Can you work these out from the model? Positions are in its coordinate system, mm. A direction names the side the tool comes from. Coordinates: 2 decimals unless noted, no trailing zeros. Write each loop counter-clockwise with the first axis right and the second up, starting at its lowest first coordinate (ties: lowest second). Pieces come first, ordered by that corner, then holes. Notation, with made-up numbers: M 8.25,51 L 13.25,51 A10 ccw 13.25,63 Z; hole C 48,-3.75 d10. An arc over 180 degrees is marked long. Use one line per item in the form item = value. Start each with the question number.
```python
from build123d import *

# Parameters (mm, degrees)
SKETCH003_R   = 292.1
SKETCH003_R_2 = 6.35
PAD003_DEPTH  = 19.05
SKETCH004_R   = 38.1
PAD004_DEPTH  = 31.75
SKETCH005_W   = 25.4
SKETCH005_H   = 25.4
PAD005_DEPTH  = 3.175


with BuildPart() as part:
    # Sketch003 → Pad003 (new body)
    with BuildSketch(Plane.XY):
        Circle(SKETCH003_R)
        Circle(SKETCH003_R_2, mode=Mode.SUBTRACT)
    extrude(amount=PAD003_DEPTH)

    # Sketch004 (on Face3 of Pad003) → Pad004 (join)
    with BuildSketch(Plane(origin=(0, 0, 0), x_dir=(1, 0, 0), z_dir=(0, 0, -1))):
        with Locations((0, 279.4)):
            Circle(SKETCH004_R)
        with Locations((241.967498, -139.7)):
            Circle(SKETCH004_R)
        with Locations((-241.967498, -139.7)):
            Circle(SKETCH004_R)
    extrude(amount=PAD004_DEPTH)

    # Sketch005 (on Face6 of Pad004) → Pad005 (join)
    with BuildSketch(Plane.XY.offset(19.05)):
        Polygon((-237.318975, 122.351477), (-224.618975, 144.348523), (-246.61602, 157.048523), (-259.31602, 135.051477), align=None)
        Polygon((237.318975, 122.351477), (259.31602, 135.051477), (246.61602, 157.048523), (224.618975, 144.348523), align=None)
        with Locations((0, -279.4)):
            Rectangle(SKETCH005_W, SKETCH005_H)
    extrude(amount=PAD005_DEPTH)


solid = part.part
```
1) Suppose I cut it at A-A on z = -20. Please give me the cut outline in (x, y), and give its area (3 significant figures).
2) Please list where these lines run through material, in increasing order: line 1 (Y direction, x = 0, z = 10); line 2 (Z direction, x = -117, y = -21.5); line 3 (X direction, y = -268.5, z = -6.5).
3) Will these pins go through, and if not, where does the flat tip stop? pin 1 Ø23.5 at (x, y) = (-267, 159.5) entering from +Z; pin 2 Ø1.6 at (y, z) = (-280, 20.5) entering from +X; pin 3 Ø6 at (x, y) = (118, -191) entering from -Z; pin 4 Ø7.5 at (x, y) = (0, 0) entering from -Z.
4) If we mould it in two halves opening along X, with no side actions, what happens to faces 1 (the face through (-272.202, 162.883, -15.653)), 2 (the face through (-248.47, 128.79, 20.62)), 3 (the face through (0, -279, 22.225))? For each: +X half, -X half, draft (parallel to the pull), parting line (faces both ways), or undercut.
5) Suppose I cut it at C-C on x = -172.5. Please give me the cut outline in (y, z).
6) Suppose I cut it at D-D on y = 17.5. Please give me the cut outline in (x, z), and give its area (3 significant figures).
7) Suppose I cut it at B-B on y = -279.4. Please give me the cut outline in (x, z) (3 decimals), and give its area (3 significant figures).
8) Which directions (+Z, -Z, +X, -X, +Y, -Y) give clear straight access to the entire face, cutting with the end or side of a thin tool? Please do faces 4 (the face through (253.055, 145.896, 20.615)), 5 (the face through (248.16, 128.61, 20.62)), 6 (the face through (-235.464, 150.61, 20.615)), 7 (the face through (-4.1, 5.2, 0)), 8 (the face through (-231.058, 133.196, 20.615)).
Computed values:
q1.outline = C -241.97,139.7 d76.2; C 0,-279.4 d76.2; C 241.97,139.7 d76.2
q1.area = 13,700 mm²
q2.line_1 = -292.1 to -6.35, 6.35 to 292.1
q2.line_2 = 0 to 19.05
q2.line_3 = -36.51 to 36.51
q3.pin_1 = 0
q3.pin_2 = 12.7
q3.pin_3 = 0
q3.pin_4 = through
q4.face_1 = undercut
q4.face_2 = -X half
q4.face_3 = draft
q5.outline = M -235.72,0 L 235.72,0 L 235.72,19.05 L -235.72,19.05 Z
q6.outline = M -291.58,0 L 291.58,0 L 291.58,19.05 L -291.58,19.05 Z
q6.area = 11,100 mm²
q7.outline = M -85.194,0 L -38.1,0 L -38.1,-31.75 L 38.1,-31.75 L 38.1,0 L 85.194,0 L 85.194,19.05 L 12.7,19.05 L 12.7,22.225 L -12.7,22.225 L -12.7,19.05 L -85.194,19.05 Z
q7.area = 5,750 mm²
q8.face_4 = +Z, +X, +Y
q8.face_5 = +Z, +X, -Y
q8.face_6 = +Z, +Y
q8.face_7 = -Z
q8.face_8 = +Z, -Y
